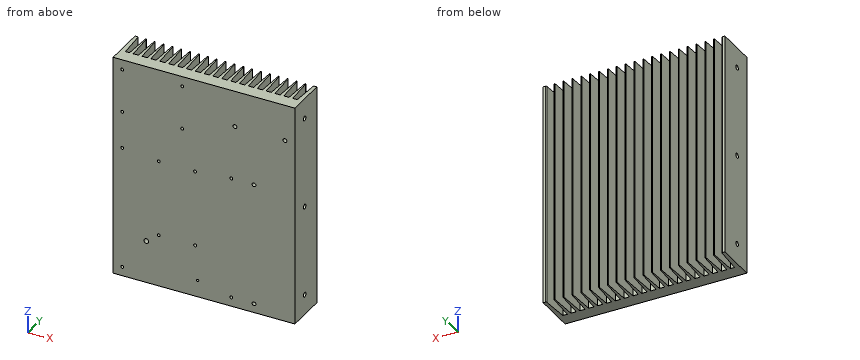
```python
from build123d import *

# Parameters (mm, degrees)
EXTRUDE_1_DEPTH       = 245
EXTRUDE_3_DEPTH       = 245
PATTERN_CURVE_1_COUNT = 19
PATTERN_CURVE_1_PITCH = 9.75
SKETCH_7_R            = 2.6
CUT_EXTRUDE_4_DEPTH   = 6
SKETCH_8_R            = 4.5
SKETCH_8_R_2          = 3.4
CUT_EXTRUDE_5_DEPTH   = 6
CUT_EXTRUDE_START     = -6
SKETCH_9_R            = 2.6
CUT_EXTRUDE_6_DEPTH   = 6
EXTRUDE_4_REACH       = 321.453
SKETCH_11_R           = 2.6
EXTRUDE_5_REACH       = 321.453
SKETCH_12_R           = 4.5
SKETCH_12_R_2         = 3.4
SKETCH_19_R           = 2.6
CUT_EXTRUDE_12_DEPTH  = 8
SKETCH_21_R           = 2.6
SKETCH_21_R_2         = 1.6
SKETCH_21_R_3         = 1.3
SKETCH_21_R_4         = 2.1
CUT_EXTRUDE_13_DEPTH  = 10


with BuildPart() as part:
    # Эскиз1 → Вытянуть1 (new body)
    with BuildSketch(Plane.XY):
        with BuildLine():
            Line((0, 45), (2.564446908, 45))
            ThreePointArc((2.564446908, 45), (3.247630994, 44.730246195), (3.562232066, 44.066519011))
            Line((3.562232066, 44.066519011), (5.5, 15))
            Line((5.5, 15), (194.5, 15))
            Line((194.5, 15), (196.437767934, 44.066519011))
            ThreePointArc((196.437767934, 44.066519011), (196.752369006, 44.730246195), (197.435553092, 45))
            Line((197.435553092, 45), (200, 45))
            Line((200, 45), (200, 0))
            Line((200, 0), (0, 0))
            Line((0, 0), (0, 45))
        make_face()
    extrude(amount=EXTRUDE_1_DEPTH)

    # Эскиз2 → Вытянуть3 (add)
    with BuildSketch(Plane.XY.offset(245)):
        with BuildLine():
            Line((11.5, 44.5), (10, 15))
            Line((10, 15), (14, 15))
            Line((14, 15), (12.5, 44.5))
            ThreePointArc((12.5, 44.5), (12, 45), (11.5, 44.5))
        make_face()
    extrude_3 = extrude(amount=-EXTRUDE_3_DEPTH)

    # Кривая1: Вытянуть3 ×19
    with Locations(*[(i * PATTERN_CURVE_1_PITCH, 0, 0) for i in range(1, PATTERN_CURVE_1_COUNT)]):
        add(extrude_3)

    # Эскиз7 → Вырез-Вытянуть4 (cut)
    with BuildSketch(Plane.ZY):
        with Locations(Location((22.5, 20, 0), (0, 0, 270))):
            Circle(SKETCH_7_R)
        with Locations(Location((222.5, 20, 0), (0, 0, 270))):
            Circle(SKETCH_7_R)
        with Locations(Location((122.5, 20, 0), (0, 0, 270))):
            Circle(SKETCH_7_R)
    extrude(amount=-CUT_EXTRUDE_4_DEPTH, mode=Mode.SUBTRACT)

    # Эскиз8 → Вырез-Вытянуть5 (cut)
    with BuildSketch(Plane(origin=(200, 0, 0), x_dir=(0, 0, -1), z_dir=(1, 0, 0))):
        with Locations((-80, 30)):
            Circle(SKETCH_8_R)
        with Locations((-165, 30)):
            Circle(SKETCH_8_R_2)
    extrude(amount=-CUT_EXTRUDE_5_DEPTH, mode=Mode.SUBTRACT)

    # Эскиз9 → Вырез-Вытянуть6 (cut)
    with BuildSketch(Plane(origin=(200, 0, 0), x_dir=(0, 0, -1), z_dir=(1, 0, 0)).offset(CUT_EXTRUDE_START)):
        with Locations(Location((-22.5, 20, 0), (0, 0, 270))):
            Circle(SKETCH_9_R)
        with Locations(Location((-122.5, 20, 0), (0, 0, 270))):
            Circle(SKETCH_9_R)
        with Locations(Location((-222.5, 20, 0), (0, 0, 270))):
            Circle(SKETCH_9_R)
    extrude(amount=CUT_EXTRUDE_6_DEPTH, mode=Mode.SUBTRACT)

    # Вытянуть4: up to this face of the body (flat: up to its plane)
    extrude_4_end = Plane(part.part.faces().sort_by_distance((4.525378677, 29.61931985, 122.5))[0])
    # Эскиз11 → Вытянуть4 (add, up to the picked face)
    with BuildSketch(Plane.ZY, mode=Mode.PRIVATE) as extrude_4_sk1:
        with Locations(Location((22.5, 20, 0), (0, 0, 180))):
            Circle(SKETCH_11_R)
    extrude_4_tool1 = split(extrude(extrude_4_sk1.sketch, amount=-EXTRUDE_4_REACH, mode=Mode.PRIVATE), bisect_by=extrude_4_end, keep=Keep.BOTH, mode=Mode.PRIVATE)
    # Эскиз11 → Вытянуть4 (add, up to the picked face)
    with BuildSketch(Plane.ZY, mode=Mode.PRIVATE) as extrude_4_sk2:
        with Locations(Location((122.5, 20, 0), (0, 0, 180))):
            Circle(SKETCH_11_R)
    extrude_4_tool2 = split(extrude(extrude_4_sk2.sketch, amount=-EXTRUDE_4_REACH, mode=Mode.PRIVATE), bisect_by=extrude_4_end, keep=Keep.BOTH, mode=Mode.PRIVATE)
    # Эскиз11 → Вытянуть4 (add, up to the picked face)
    with BuildSketch(Plane.ZY, mode=Mode.PRIVATE) as extrude_4_sk3:
        with Locations(Location((222.5, 20, 0), (0, 0, 180))):
            Circle(SKETCH_11_R)
    extrude_4_tool3 = split(extrude(extrude_4_sk3.sketch, amount=-EXTRUDE_4_REACH, mode=Mode.PRIVATE), bisect_by=extrude_4_end, keep=Keep.BOTH, mode=Mode.PRIVATE)
    add(extrude_4_tool1.solids().sort_by(Axis((0, 20, 22.5), (1, 0, 0)))[0])
    add(extrude_4_tool2.solids().sort_by(Axis((0, 20, 122.5), (1, 0, 0)))[0])
    add(extrude_4_tool3.solids().sort_by(Axis((0, 20, 222.5), (1, 0, 0)))[0])

    # Вытянуть5: up to this face of the body (flat: up to its plane)
    extrude_5_end = Plane(part.part.faces().sort_by_distance((195.474256805, 29.613852069, 122.666761542))[0])
    # Эскиз12 → Вытянуть5 (add, up to the picked face)
    with BuildSketch(Plane(origin=(200, 0, 0), x_dir=(0, 0, -1), z_dir=(1, 0, 0)), mode=Mode.PRIVATE) as extrude_5_sk1:
        with Locations((-80, 30)):
            Circle(SKETCH_12_R)
    extrude_5_tool1 = split(extrude(extrude_5_sk1.sketch, amount=-EXTRUDE_5_REACH, mode=Mode.PRIVATE), bisect_by=extrude_5_end, keep=Keep.BOTH, mode=Mode.PRIVATE)
    # Эскиз12 → Вытянуть5 (add, up to the picked face)
    with BuildSketch(Plane(origin=(200, 0, 0), x_dir=(0, 0, -1), z_dir=(1, 0, 0)), mode=Mode.PRIVATE) as extrude_5_sk2:
        with Locations((-165, 30)):
            Circle(SKETCH_12_R_2)
    extrude_5_tool2 = split(extrude(extrude_5_sk2.sketch, amount=-EXTRUDE_5_REACH, mode=Mode.PRIVATE), bisect_by=extrude_5_end, keep=Keep.BOTH, mode=Mode.PRIVATE)
    add(extrude_5_tool1.solids().sort_by(Axis((200, 30, 80), (-1, 0, 0)))[0])
    add(extrude_5_tool2.solids().sort_by(Axis((200, 30, 165), (-1, 0, 0)))[0])

    # Эскиз19 → Вырез-Вытянуть12 (cut)
    with BuildSketch(Plane.ZY):
        with Locations(Location((222.5, 20, 0), (0, 0, 180))):
            Circle(SKETCH_19_R)
        with Locations(Location((122.5, 20, 0), (0, 0, 180))):
            Circle(SKETCH_19_R)
        with Locations(Location((22.5, 20, 0), (0, 0, 180))):
            Circle(SKETCH_19_R)
    extrude(amount=-CUT_EXTRUDE_12_DEPTH, mode=Mode.SUBTRACT)

    # Эскиз21 → Вырез-Вытянуть13 (cut)
    with BuildSketch(Plane.XZ):
        with Locations((36.5, 47)):
            Circle(SKETCH_21_R)
        with Locations((10, 145)):
            Circle(SKETCH_21_R_2)
        with Locations((10, 10)):
            Circle(SKETCH_21_R_2)
        with Locations((130, 10)):
            Circle(SKETCH_21_R_2)
        with Locations((130, 145)):
            Circle(SKETCH_21_R_2)
        with Locations((50.25, 141.4)):
            Circle(SKETCH_21_R_2)
        with Locations((90.25, 141.4)):
            Circle(SKETCH_21_R_2)
        with Locations((50.25, 57.6)):
            Circle(SKETCH_21_R_2)
        with Locations((90.25, 57.6)):
            Circle(SKETCH_21_R_2)
        with Locations((93, 18.5)):
            Circle(SKETCH_21_R_3)
        with Locations((134, 205)):
            Circle(SKETCH_21_R_4)
        with Locations((155, 145)):
            Circle(SKETCH_21_R_4)
        with Locations((189, 205)):
            Circle(SKETCH_21_R_4)
        with Locations((155, 10)):
            Circle(SKETCH_21_R_4)
        with Locations((76, 234)):
            Circle(SKETCH_21_R_2)
        with Locations((10, 234)):
            Circle(SKETCH_21_R_2)
        with Locations((10, 186)):
            Circle(SKETCH_21_R_2)
        with Locations((76, 186)):
            Circle(SKETCH_21_R_2)
    extrude(amount=-CUT_EXTRUDE_13_DEPTH, mode=Mode.SUBTRACT)


solid = part.part
```
Source: CAD feature listing. Evaluate the final solid. Frame: model axes, mm. Coordinates: 2 decimals unless noted, no trailing zeros. Return JSON: item names as keys, results as strings. Group by question number.
1) Section query A-A, the plane y = 34. State how many separate pieces and enclosed holes the cut face has, plus the area to 3 significant figures.
2) Ray query, line 1 along X through (y, z) = (3, 145); line 2 along Z through (x, y) = (10, 2.75); line 3 along Z through (x, y) = (76, 6). Return the intervals inside material, ascending.
3) Contact query for flat-ended pins moving along their axis: P1, Ø3.5, axis at x = 10, z = 145, coming from the +Y side; P2, Ø3, axis at x = 17.5, z = 96.5, coming from the +Y side; P3, Ø1.9, axis at x = 76, z = 186, coming from the -Y side. Output: stop coordinate, or through.
From the geometry:
{
 "1": {"separate pieces": "21", "enclosed holes": "0", "area": "11,700 mm²"},
 "2": {"line 1": "0 to 8.4, 11.6 to 128.4, 131.6 to 152.9, 157.1 to 200", "line 2": "0 to 8.4, 11.6 to 143.4, 146.6 to 184.4, 187.6 to 232.4, 235.6 to 245", "line 3": "0 to 184.4, 187.6 to 232.4, 235.6 to 245"},
 "3": {"P1": "y = 44.93", "P2": "y = 15", "P3": "y = 10"}
}
